Check sheet for the modelled part. Datum: model origin and axes. Units: mm. Face numbers are marked on the shaded views. A direction names the side the tool comes from. Give positions to 0.01 mm unless a question says otherwise; leave off trailing zeros. Order: outer loops, then holes, each group sorted by start corner. A loop starts at its lowest first (then second) coordinate and runs counter-clockwise, first axis right, second up.
Item 1: Sectioned sample at B-B on x = 10. Record the boundary of the cut face in (y, z).
Item 2: Gauge pin test, flat ends, axial feed: P1, Ø8, axis at x = 21.5, z = -20.5, coming from the +Y side; P2, Ø1.6, axis at x = 10, z = -30, coming from the -Y side. Record the tip position at first contact, or that the pin passes through.
Item 3: Sectioned sample at A-A on z = 30. Record the boundary of the cut face in (x, y), and give its area (3 significant figures).
Item 4: Sectioned sample at C-C on y = 3.25. Record the boundary of the cut face in (x, z), and give its area (3 significant figures).
Item 5: Sectioned sample at D-D on x = -30. Record the boundary of the cut face in (y, z), and give its area (3 significant figures).
Item 6: Material ranges on line 1 along X through (y, z) = (0.7, 20); line 2 along Y through (x, z) = (29.5, -14.5); line 3 along Y through (x, z) = (-29.5, 36.5), recorded low to high.
Item 7: Access from +Z, -Z, +X, -X, +Y, -Y to the whole of each face (thin tool, end or side, straight path). Record for the marked faces 1 and 2.
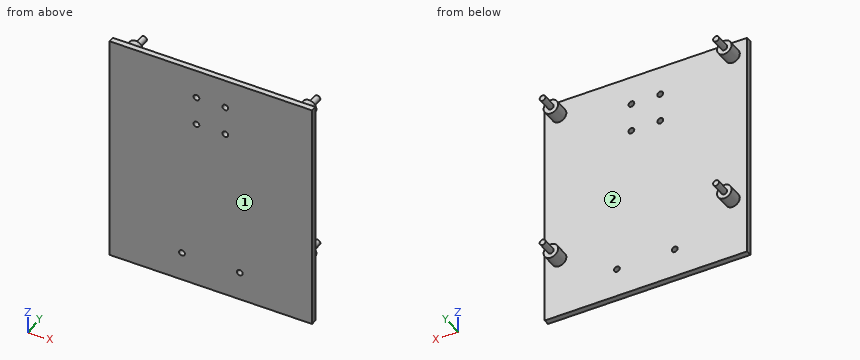
from build123d import *

# Parameters (mm, degrees)
BOSS_EXTRUDE1_OUTLINE_W = 70
BOSS_EXTRUDE1_OUTLINE_H = 80
BOSS_EXTRUDE1_DEPTH     = 2
SKETCH2_R               = 2.5
BOSS_EXTRUDE2_DEPTH     = 5
SKETCH3_R               = 1
BOSS_EXTRUDE3_DEPTH     = 5
SKETCH4_R               = 1
CUT_EXTRUDE1_DEPTH      = 55.083269132
SKETCH5_R               = 1
CUT_EXTRUDE2_DEPTH      = 55.083269132


# Read off the part's stored shape, not the designer's step: Boss-Extrude1
with BuildPart() as part:
    # Boss-Extrude1 outline → Boss-Extrude1 (new body)
    with BuildSketch(Plane(origin=(0, 0, 0), x_dir=(1, 0, 0), z_dir=(0, 1, 0))):
        Rectangle(BOSS_EXTRUDE1_OUTLINE_W, BOSS_EXTRUDE1_OUTLINE_H)
    extrude(amount=BOSS_EXTRUDE1_DEPTH)

    # Sketch2 → Boss-Extrude2 (add)
    with BuildSketch(Plane(origin=(0, 2, 0), x_dir=(1, 0, 0), z_dir=(0, 1, 0))):
        with Locations(Location((-30, 19, 0), (0, 0, 270))):
            Circle(SKETCH2_R)
        with Locations(Location((30, 19, 0), (0, 0, 270))):
            Circle(SKETCH2_R)
        with Locations(Location((-30, -35, 0), (0, 0, 270))):
            Circle(SKETCH2_R)
        with Locations(Location((30, -35, 0), (0, 0, 270))):
            Circle(SKETCH2_R)
    extrude(amount=BOSS_EXTRUDE2_DEPTH)

    # Sketch3 → Boss-Extrude3 (add)
    with BuildSketch(Plane(origin=(0, 7, 0), x_dir=(1, 0, 0), z_dir=(0, 1, 0))):
        with Locations(Location((-30, 19, 0), (0, 0, 270))):
            Circle(SKETCH3_R)
        with Locations(Location((30, 19, 0), (0, 0, 270))):
            Circle(SKETCH3_R)
        with Locations(Location((30, -35, 0), (0, 0, 270))):
            Circle(SKETCH3_R)
        with Locations(Location((-30, -35, 0), (0, 0, 270))):
            Circle(SKETCH3_R)
    extrude(amount=BOSS_EXTRUDE3_DEPTH)

    # Sketch4 → Cut-Extrude1 (cut, through all)
    with BuildSketch(Plane(origin=(0, 2, 0), x_dir=(1, 0, 0), z_dir=(0, 1, 0))):
        with Locations(Location((-5, -30, 0), (0, 0, 270))):
            Circle(SKETCH4_R)
        with Locations(Location((-5, -20, 0), (0, 0, 270))):
            Circle(SKETCH4_R)
        with Locations(Location((5, -20, 0), (0, 0, 270))):
            Circle(SKETCH4_R)
        with Locations(Location((5, -30, 0), (0, 0, 270))):
            Circle(SKETCH4_R)
    extrude(amount=-CUT_EXTRUDE1_DEPTH, mode=Mode.SUBTRACT)

    # Sketch5 → Cut-Extrude2 (cut, through all)
    with BuildSketch(Plane(origin=(0, 2, 0), x_dir=(1, 0, 0), z_dir=(0, 1, 0))):
        with Locations(Location((-10, 30, 0), (0, 0, 270))):
            Circle(SKETCH5_R)
        with Locations(Location((10, 30, 0), (0, 0, 270))):
            Circle(SKETCH5_R)
    extrude(amount=-CUT_EXTRUDE2_DEPTH, mode=Mode.SUBTRACT)


solid = part.part
Report:
1. outline: (0, -40) - (2, -40) - (2, -31) - (0, -31) - close; (0, -29) - (2, -29) - (2, 40) - (0, 40) - close
2. P1: stops at y = 2
2. P2: passes through
3. outline: (-35, 0) - (-6, 0) - (-6, 2) - (-35, 2) - close; (-4, 0) - (4, 0) - (4, 2) - (-4, 2) - close; (6, 0) - (35, 0) - (35, 2) - (6, 2) - close
3. area: 132 mm2
4. outline: circle Ø5 at (-30, -19); circle Ø5 at (-30, 35); circle Ø5 at (30, -19); circle Ø5 at (30, 35)
4. area: 78.5 mm2
5. outline: (0, -40) - (2, -40) - (2, -21.5) - (7, -21.5) - (7, -20) - (12, -20) - (12, -18) - (7, -18) - (7, -16.5) - (2, -16.5) - (2, 32.5) - (7, 32.5) - (7, 34) - (12, 34) - (12, 36) - (7, 36) - (7, 37.5) - (2, 37.5) - (2, 40) - (0, 40) - close
5. area: 230 mm2
6. line 1: x = -35 to -6, -4 to 4, 6 to 35
6. line 2: y = 0 to 2
6. line 3: y = 0 to 7
7. face 1: +Z, -Z, +X, -X, -Y
7. face 2: +Y
